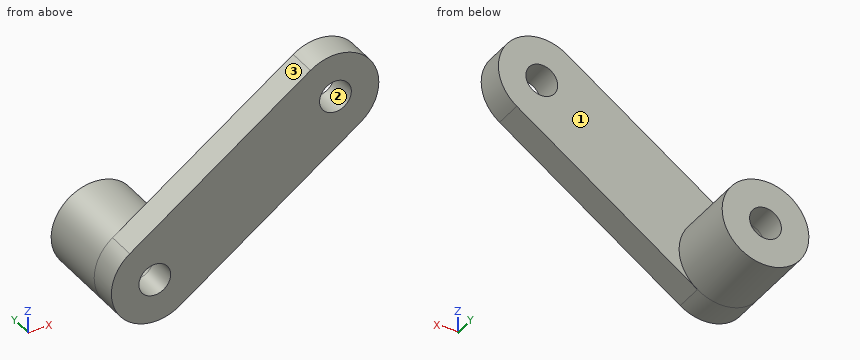
```python
from build123d import *
from build123d.topology import SkipClean

# Parameters (mm, degrees)
BOSS_EXTRUDE1_DEPTH = 2
SKETCH2_R           = 3
SKETCH2_R_2         = 1.1
BOSS_EXTRUDE2_DEPTH = 5
SKETCH4_R           = 1.1
CUT_EXTRUDE1_DEPTH  = 5


with BuildPart() as part:
    # Sketch1 → Boss-Extrude1 (new body)
    with BuildSketch(Plane(origin=(0, 0, 0), x_dir=(1, 0, 0), z_dir=(0, 1, 0))):
        with BuildLine():
            Line((-15.769757973, 16.275767743), (-3.269757973, 7.450767743))
            ThreePointArc((-3.269757973, 7.450767743), (-2.549232257, 3.269757973), (-6.730242027, 2.549232257))
            Line((-6.730242027, 2.549232257), (-19.230242027, 11.374232257))
            ThreePointArc((-19.230242027, 11.374232257), (-19.950767743, 15.555242027), (-15.769757973, 16.275767743))
        make_face()
    extrude(amount=BOSS_EXTRUDE1_DEPTH)

    # Sketch2 → Boss-Extrude2 (add)
    with SkipClean():  # the faces are left unmerged after this step: merging them gives an invalid solid
        with BuildSketch(Plane(origin=(0, 2, 0), x_dir=(1, 0, 0), z_dir=(0, 1, 0))):
            with Locations(Location((-17.5, 13.825, 0), (0, 0, 54.777908305))):
                Circle(SKETCH2_R)
            with Locations(Location((-17.5, 13.825, 0), (0, 0, 270))):
                Circle(SKETCH2_R_2, mode=Mode.SUBTRACT)
        extrude(amount=BOSS_EXTRUDE2_DEPTH)
    add(part.part.scale(1), mode=Mode.REPLACE)  # the faces are merged on a copy

    # Sketch4 → Cut-Extrude1 (cut)
    with BuildSketch(Plane.XZ):
        with Locations(Location((-5, -5, 0), (0, 0, 270))):
            Circle(SKETCH4_R)
        with Locations(Location((-17.5, -13.825, 0), (0, 0, 270))):
            Circle(SKETCH4_R)
    extrude(amount=-CUT_EXTRUDE1_DEPTH, mode=Mode.SUBTRACT)


solid = part.part
```
Can you work these out from the model? Positions are in its coordinate system, mm. Face numbers are marked on the shaded views. Coordinates: 2 decimals unless noted, no trailing zeros. Loops run counter-clockwise (first coordinate to the right, second up) from the corner with the lowest first, then second, coordinate; pieces in that order, holes last. Notation, with made-up numbers: (-15, -12) - (-3, -12) arc R15 ccw to (-3, -6) - close; hole circle Ø4 at (17, -4.5). An arc over 180 degrees is marked (long way). Answer as CSV lines item,"result". Start each with the question number.
1) Suppose I cut it at B-B (z = -14.5). Please give me the cut outline in (x, y).
2) Suppose I cut it at D-D (x = -15). Please give me the cut outline in (y, z), plus the area to 3 significant figures.
3) Suppose I cut it at C-C (y = 2.5). Please give me the cut outline in (x, z) (3 decimals), plus the area to 3 significant figures.
4) For pin 1 (1 mm diameter, centred on y = 2, z = -14.5, fed in from -X); pin 2 (1.5 mm diameter, centred on x = -14.5, y = 4, fed in from +Z); pin 3 (6 mm diameter, centred on x = -14, z = -8.5, fed in from +Y); pin 4 (1.8 mm diameter, centred on x = -17.5, z = -13.825, fed in from -Y), each with a flat end and sliding along its axis, tell me the tip position at first contact or that it passes through.
5) Suppose I cut it at A-A (x = -17.75). Please give me the cut outline in (y, z).
6) I need wall thicknesses on line 1 (Y direction, x = -12.75, z = -11.5); line 2 (Z direction, x = -17.5, y = 0.6) (3 decimals); line 3 (Z direction, x = -16.75, y = 4). Which ranges of each line are inside material? Lowest first, please. Write a range as from..to.
7) Thinking about a two-plate mould opening in Z: for the marked faces 1, 2 and 3, which applies, pulls with the +Z half, pulls with the -Z half, needs draft (parallel to the pull), parting line crosses it, or undercut?
Check result:
1,outline,"(-20.42, 0) - (-18.37, 0) - (-18.37, 7) - (-20.42, 7) - close; (-16.63, 0) - (-13.25, 0) - (-13.25, 2) - (-14.58, 2) - (-14.58, 7) - (-16.63, 7) - close"
2,outline,"(0, -15.73) - (2, -15.73) - (2, -15.48) - (7, -15.48) - (7, -12.17) - (2, -12.17) - (2, -8.39) - (0, -8.39) - close"
2,area,"31.3 mm²"
3,outline,"circle Ø6 at (-17.5, -13.825); hole circle Ø2.2 at (-17.5, -13.825)"
3,area,"24.5 mm²"
4,pin 1,"stops at x = -20.49"
4,pin 2,"stops at z = -11.84"
4,pin 3,"stops at y = 2"
4,pin 4,"passes through"
5,outline,"(0, -16.81) - (7, -16.81) - (7, -14.9) - (0, -14.9) - close; (0, -12.75) - (7, -12.75) - (7, -10.84) - (2, -10.84) - (2, -10.33) - (0, -10.33) - close"
6,line 1,"y = 0..2"
6,line 2,"z = -16.825..-14.925, -12.725..-10.153"
6,line 3,"z = -16.73..-14.63, -13.02..-10.92"
7,face 1,"needs draft"
7,face 2,"undercut"
7,face 3,"pulls with the +Z half"
